Source: three-view drawing plus pictorial views. Frame: mm from the lowest corner of the part. Give positions to 0.01 mm unless a question says otherwise; leave off trailing zeros. Write each loop counter-clockwise with the first axis right and the second up, starting at its lowest first coordinate (ties: lowest second). Pieces come first, ordered by that corner, then holes. Notation, with made-up numbers: (27, 1) -> (74, 1) arc R35 cw to (74, 38) -> close; hole circle Ø1 at (5.25, 36). An arc over 180 degrees is marked (long way). Answer in a Markdown table with one row per item. Add a question column.
Item 1: First-contact query: P1, Ø1.9, axis at x = 381, y = 3, coming from the -Z side. Flat tip, straight axial feed; report the tip coordinate or a pass-through.
Item 2: Material intervals for probe 1 along X at (y, z) = (2.75, 19) (3 decimals); probe 2 along Z at (x, y) = (438, 1.5), sorted ascending. Write a range as from..to.
Item 3: Section query C-C on x = 448. Output: boundary loops of the cut face in (y, z).
Item 4: Section query A-A on z = 24.5. Output: boundary loops of the cut face in (x, y) (3 decimals), plus the area to 3 significant figures.
Item 5: Section query B-B on y = 2. Output: boundary loops of the cut face in (x, z) (3 decimals), plus the area to 3 significant figures.
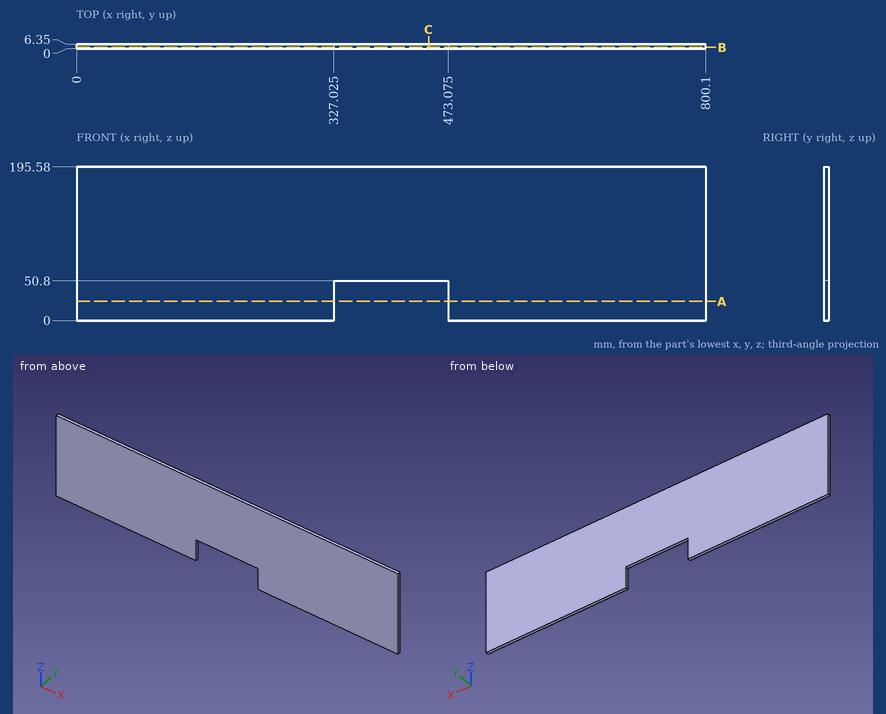
Findings below:
| question | item | result |
|---|---|---|
| 1 | P1 | stops at z = 50.8 |
| 2 | probe 1 | x = 0..327.025, 473.075..800.1 |
| 2 | probe 2 | z = 50.8..195.58 |
| 3 | outline | (0, 50.8) -> (6.35, 50.8) -> (6.35, 195.58) -> (0, 195.58) -> close |
| 4 | outline | (0, 0) -> (327.025, 0) -> (327.025, 6.35) -> (0, 6.35) -> close; (473.075, 0) -> (800.1, 0) -> (800.1, 6.35) -> (473.075, 6.35) -> close |
| 4 | area | 4,150 mm^2 |
| 5 | outline | (0, 0) -> (327.025, 0) -> (327.025, 50.8) -> (473.075, 50.8) -> (473.075, 0) -> (800.1, 0) -> (800.1, 195.58) -> (0, 195.58) -> close |
| 5 | area | 149,000 mm^2 |
